from build123d import *

# Parameters (mm, degrees)
F0_W     = 76.2
F0_H     = 76.2
F1_DEPTH = 38.1
F3_W     = 25.4
F3_H     = 25.4
F4_DEPTH = 76.201


with BuildPart() as f1:
    # F0 (on Front) → F1 (new body, symmetric)
    with BuildSketch(Plane.XZ):
        Rectangle(F0_W, F0_H)
    extrude(amount=F1_DEPTH, both=True)

    # F3 (on face) → F4 (cut, through all)
    with BuildSketch(Plane.XZ.offset(38.1)):
        Rectangle(F3_W, F3_H)
    extrude(amount=-F4_DEPTH, mode=Mode.SUBTRACT)


solid = f1.part
Build history of the part. All positions in model axes, mm. A direction names the side the tool comes from. Coordinates: 2 decimals unless noted, no trailing zeros. Write each loop counter-clockwise with the first axis right and the second up, starting at its lowest first coordinate (ties: lowest second). Pieces come first, ordered by that corner, then holes.
(1) Cut at C-C on z = -5. List the corners of the cut face in (x, y), and give its area (3 significant figures).
(2) Drill centre line: line 1 (Z direction, x = 1, y = 5). Where is it in solid material? Low to high.
(3) Cut at A-A on x = -10. List the corners of the cut face in (y, z).
(4) Cut at B-B on y = 9. List the corners of the cut face in (x, z).
(5) Mould opens along Z. For faces 1 (the flat face through (-1, -1, -38.1)), 2 (the flat face through (0, -1, 12.7)), 3 (the flat face through (16, -38.1, 1)), 4 (the flat face through (0, -1, -12.7)) say: pulls with the +Z half, pulls with the -Z half, needs draft (parallel to the pull), parting line crosses it, or undercut.
(6) 3-axis set-ups, long thin cutter, end or side, ignore diameter. For faces 5 (the flat face through (12.7, -1, 0)), 6 (the flat face through (-1, -1, 38.1)): which of +Z, -Z, +X, -X, +Y, -Y reach the whole face in a straight line?
Working result:
1. outline: (-38.1, -38.1) - (-12.7, -38.1) - (-12.7, 38.1) - (-38.1, 38.1) - close; (12.7, -38.1) - (38.1, -38.1) - (38.1, 38.1) - (12.7, 38.1) - close
1. area: 3,870 mm2
2. line 1: z = -38.1 to -12.7, 12.7 to 38.1
3. outline: (-38.1, -38.1) - (38.1, -38.1) - (38.1, -12.7) - (-38.1, -12.7) - close; (-38.1, 12.7) - (38.1, 12.7) - (38.1, 38.1) - (-38.1, 38.1) - close
4. outline: (-38.1, -38.1) - (38.1, -38.1) - (38.1, 38.1) - (-38.1, 38.1) - close; hole (-12.7, -12.7) - (12.7, -12.7) - (12.7, 12.7) - (-12.7, 12.7) - close
5. face 1: pulls with the -Z half
5. face 2: undercut
5. face 3: needs draft
5. face 4: undercut
6. face 5: +Y, -Y
6. face 6: +Z, +X, -X, +Y, -Y
